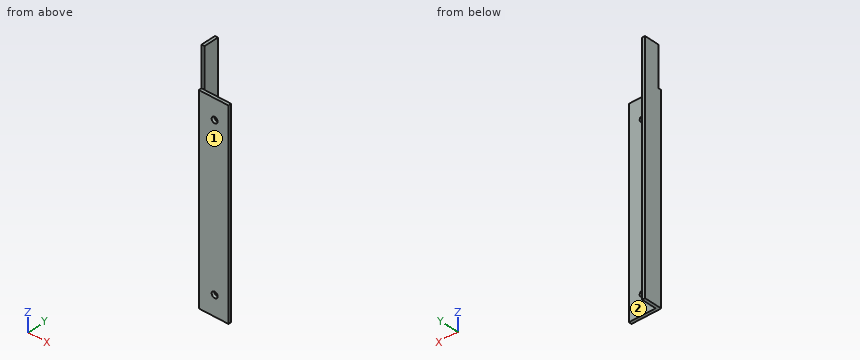
```python
from build123d import *

# Parameters (mm, degrees)
EXTRUSION1_DEPTH = 100
ESQUISSE2_R      = 1.5
EXTRUSION2_DEPTH = 120
ESQUISSE3_W      = 1.5
ESQUISSE3_H      = 7.5
EXTRUSION3_DEPTH = 20


with BuildPart() as part:
    # Esquisse1 → Extrusion1 (new body)
    with BuildSketch(Plane.XY):
        Polygon((-18.340739011, -0.545052632), (-18.340739011, -9.545052632), (-3.340739011, -9.545052632), (-3.340739011, -8.045052632), (-16.840739011, -8.045052632), (-16.840739011, -0.545052632), align=None)
    extrude(amount=EXTRUSION1_DEPTH)

    # Esquisse2 → Extrusion2 (cut)
    with BuildSketch(Plane(origin=(0, -8.045052632, 0), x_dir=(-1, 0, 0), z_dir=(0, 1, 0))):
        with Locations((10.340739011, 90)):
            Circle(ESQUISSE2_R)
        with Locations((10.340739011, 10)):
            Circle(ESQUISSE2_R)
    extrude(amount=-EXTRUSION2_DEPTH, mode=Mode.SUBTRACT)

    # Esquisse3 → Extrusion3 (add)
    with BuildSketch(Plane.XY.offset(100)):
        with Locations((-17.590739011, -4.295052632)):
            Rectangle(ESQUISSE3_W, ESQUISSE3_H)
    extrude(amount=EXTRUSION3_DEPTH)


solid = part.part
```
Part model, mm, in its own coordinate system. Face numbers are marked on the shaded views. A direction names the side the tool comes from. Coordinates: 2 decimals unless noted, no trailing zeros. Write each loop counter-clockwise with the first axis right and the second up, starting at its lowest first coordinate (ties: lowest second). Pieces come first, ordered by that corner, then holes.
Item 1: Which spindle directions (+Z, -Z, +X, -X, +Y, -Y) get a long thin tool onto all of the face, cutting with end or side? Do the marked faces 1 and 2. Say none if no direction does.
Item 2: Probe line 1 (X direction, y = -8.8, z = 90); line 2 (Y direction, x = -10, z = 50.5); line 3 (X direction, y = -6.5, z = 44). List the from-to ranges inside material, lowest first.
Item 3: Slice it at C-C (z = 112). Write the cut outline in (x, y), and give its area (4 significant figures).
Item 4: Slice it at A-A (z = 90). Write the cut outline in (x, y).
Item 5: Slice it at B-B (x = -14.25). Write the cut outline in (y, z).
Item 6: Pin check, flat tips, straight feed: pin 1 (1.2 mm diameter, centred on x = -18, z = 110, fed in from -Y); pin 2 (1.6 mm diameter, centred on x = -13.5, y = -9, fed in from +Z). Stop position of each tip, or through.
Results found:
1. face 1: +Z, -Z, +X, -X, -Y
1. face 2: +Z, -Z, +X, +Y
2. line 1: x = -18.34 to -11.84, -8.84 to -3.34
2. line 2: y = -9.55 to -8.05
2. line 3: x = -18.34 to -16.84
3. outline: (-18.34, -8.05) - (-16.84, -8.05) - (-16.84, -0.55) - (-18.34, -0.55) - close
3. area: 11.25 mm2
4. outline: (-18.34, -9.55) - (-11.84, -9.55) - (-11.84, -8.05) - (-16.84, -8.05) - (-16.84, -0.55) - (-18.34, -0.55) - close; (-8.84, -9.55) - (-3.34, -9.55) - (-3.34, -8.05) - (-8.84, -8.05) - close
5. outline: (-9.55, 0) - (-8.05, 0) - (-8.05, 100) - (-9.55, 100) - close
6. pin 1: stops at y = -8.05
6. pin 2: stops at z = 100
